Model file for the job. Use its own axes, mm. Face numbers are marked on the shaded views. A direction names the side the tool comes from. Give positions to 0.01 mm unless a question says otherwise; leave off trailing zeros. Answer in a Markdown table with one row per item.
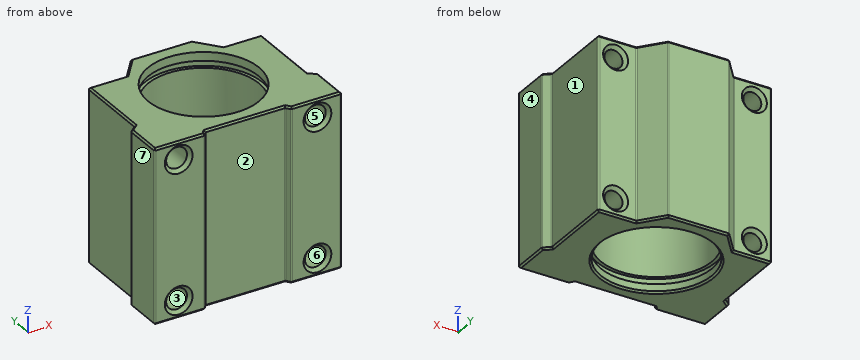
```python
from build123d import *

# Parameters (mm, degrees)
SKETCH1_R           = 16
BOSS_EXTRUDE1_DEPTH = 50
CUT_EXTRUDE1_REACH  = 72.071
SKETCH2_R           = 2.6
SKETCH3_R           = 3
CUT_EXTRUDE2_DEPTH  = 12
SKETCH4_W           = 2
SKETCH4_H           = 1
CHAMFER1_SIZE       = 1
CHAMFER2_SIZE       = 0.5
FILLET2_R           = 0.5


with BuildPart() as part:
    # Sketch1 → Boss-Extrude1 (new body)
    with BuildSketch(Plane.XY):
        Polygon((8.75, 0), (-8.75, 0), (-14, -6.5), (-25, -6.5), (-25, -28.31372549), (-27, -30), (-27, -41), (-12.5, -41), (-11.5, -39.7), (11.5, -39.7), (12.5, -41), (27, -41), (27, -30), (25, -28.31372549), (25, -6.5), (14, -6.5), align=None)
        with Locations((0, -20)):
            Circle(SKETCH1_R, mode=Mode.SUBTRACT)
    extrude(amount=BOSS_EXTRUDE1_DEPTH)

    # Sketch2 → Cut-Extrude1 (cut, up to next)
    with BuildSketch(Plane(origin=(0, 0, 0), x_dir=(1, 0, 0), z_dir=(0, 1, 0)), mode=Mode.PRIVATE) as cut_extrude1_sk1:
        with Locations(Location((-20, -45, 0), (0, 0, 270))):
            Circle(SKETCH2_R)
    cut_extrude1_tool1 = extrude(cut_extrude1_sk1.sketch, amount=-CUT_EXTRUDE1_REACH, mode=Mode.PRIVATE) & part.part
    # Sketch2 → Cut-Extrude1 (cut, up to next)
    with BuildSketch(Plane(origin=(0, 0, 0), x_dir=(1, 0, 0), z_dir=(0, 1, 0)), mode=Mode.PRIVATE) as cut_extrude1_sk2:
        with Locations(Location((20, -45, 0), (0, 0, 270))):
            Circle(SKETCH2_R)
    cut_extrude1_tool2 = extrude(cut_extrude1_sk2.sketch, amount=-CUT_EXTRUDE1_REACH, mode=Mode.PRIVATE) & part.part
    # Sketch2 → Cut-Extrude1 (cut, up to next)
    with BuildSketch(Plane(origin=(0, 0, 0), x_dir=(1, 0, 0), z_dir=(0, 1, 0)), mode=Mode.PRIVATE) as cut_extrude1_sk3:
        with Locations(Location((20, -5, 0), (0, 0, 270))):
            Circle(SKETCH2_R)
    cut_extrude1_tool3 = extrude(cut_extrude1_sk3.sketch, amount=-CUT_EXTRUDE1_REACH, mode=Mode.PRIVATE) & part.part
    # Sketch2 → Cut-Extrude1 (cut, up to next)
    with BuildSketch(Plane(origin=(0, 0, 0), x_dir=(1, 0, 0), z_dir=(0, 1, 0)), mode=Mode.PRIVATE) as cut_extrude1_sk4:
        with Locations(Location((-20, -5, 0), (0, 0, 270))):
            Circle(SKETCH2_R)
    cut_extrude1_tool4 = extrude(cut_extrude1_sk4.sketch, amount=-CUT_EXTRUDE1_REACH, mode=Mode.PRIVATE) & part.part
    add(cut_extrude1_tool1.solids().sort_by_distance((-20, 0, 45))[0], mode=Mode.SUBTRACT)
    add(cut_extrude1_tool2.solids().sort_by_distance((20, 0, 45))[0], mode=Mode.SUBTRACT)
    add(cut_extrude1_tool3.solids().sort_by_distance((20, 0, 5))[0], mode=Mode.SUBTRACT)
    add(cut_extrude1_tool4.solids().sort_by_distance((-20, 0, 5))[0], mode=Mode.SUBTRACT)

    # Sketch3 → Cut-Extrude2 (cut)
    with BuildSketch(Plane.XZ.offset(41)):
        with Locations(Location((-20, 45, 0), (0, 0, 270))):
            Circle(SKETCH3_R)
        with Locations(Location((20, 45, 0), (0, 0, 90))):
            Circle(SKETCH3_R)
        with Locations(Location((20, 5, 0), (0, 0, 270))):
            Circle(SKETCH3_R)
        with Locations(Location((-20, 5, 0), (0, 0, 90))):
            Circle(SKETCH3_R)
    extrude(amount=-CUT_EXTRUDE2_DEPTH, mode=Mode.SUBTRACT)

    # Sketch4 → Cut-Revolve1 (revolve, cut)
    with BuildSketch(Plane(origin=(0, 0, 0), x_dir=(0, 0, -1), z_dir=(1, 0, 0))):
        with Locations((-46.5, -3.5)):
            Rectangle(SKETCH4_W, SKETCH4_H)
        with Locations((-3.5, -3.5)):
            Rectangle(SKETCH4_W, SKETCH4_H)
    revolve(axis=Axis((0, -20, 0), (0, 0, 1)), mode=Mode.SUBTRACT)

    # Chamfer1
    chamfer1_edges = [part.edges().sort_by_distance(p)[0] for p in [
        (-20, -6.5, 42.4),
        (20, -6.5, 42.4),
        (20, -6.5, 2.4),
        (-20, -6.5, 2.4),
        (-20, -41, 48),
        (20, -41, 42),
        (20, -41, 8),
        (-20, -41, 2),
    ]]
    chamfer(chamfer1_edges, length=CHAMFER1_SIZE)

    # Chamfer2
    chamfer2_edges = [part.edges().sort_by_distance(p)[0] for p in [
        (0, -39.7, 50),
        (12, -40.35, 50),
        (-27, -35.5, 0),
        (-26, -29.156862745, 0),
        (-25, -17.406862745, 0),
        (-19.5, -6.5, 0),
        (-11.375, -3.25, 0),
        (19.75, -41, 50),
        (0, 0, 0),
        (11.375, -3.25, 0),
        (19.5, -6.5, 0),
        (25, -17.406862745, 0),
        (26, -29.156862745, 0),
        (27, -35.5, 0),
        (19.75, -41, 0),
        (12, -40.35, 0),
        (27, -35.5, 50),
        (0, -39.7, 0),
        (-12, -40.35, 0),
        (-19.75, -41, 0),
        (26, -29.156862745, 50),
        (25, -17.406862745, 50),
        (19.5, -6.5, 50),
        (11.375, -3.25, 50),
        (0, 0, 50),
        (-11.375, -3.25, 50),
        (-16, -20, 0),
        (-19.75, -41, 50),
        (-19.5, -6.5, 50),
        (-25, -17.406862745, 50),
        (-26, -29.156862745, 50),
        (-27, -35.5, 50),
        (-12, -40.35, 50),
    ]]
    chamfer(chamfer2_edges, length=CHAMFER2_SIZE)

    # Fillet2
    fillet2_edges = [part.edges().sort_by_distance(p)[0] for p in [
        (14, -6.5, 25),
        (25, -6.5, 25),
        (8.75, 0, 25),
        (-8.75, 0, 25),
        (-14, -6.5, 25),
        (-25, -6.5, 25),
        (-25, -28.31372549, 25),
        (-27, -30, 25),
        (-27, -41, 25),
        (-12.5, -41, 25),
        (-11.5, -39.7, 25),
        (11.5, -39.7, 25),
        (12.5, -41, 25),
        (27, -41, 25),
        (27, -30, 25),
        (25, -28.31372549, 25),
    ]]
    fillet(fillet2_edges, radius=FILLET2_R)


solid = part.part
```
(1) Which spindle directions (+Z, -Z, +X, -X, +Y, -Y) get a long thin tool onto all of the face, cutting with end or side? Do the marked faces 1, 2 and 3. Say none if no direction does.
Established:
| item | result |
|---|---|
| face 1 | +Z, -Z, +X, +Y |
| face 2 | +Z, -Z, -Y |
| face 3 | -Y |
(2) Mould opens along X. For the marked faces 4, 5, 6 and 7 say: pulls with the +X half, pulls with the -X half, needs draft (parallel to the pull), parting line crosses it, or undercut.
Established:
| item | result |
|---|---|
| face 4 | pulls with the +X half |
| face 5 | undercut |
| face 6 | undercut |
| face 7 | pulls with the -X half |
(3) Flat gauge pins, fed straight in: P1, Ø9.5, axis at x = -20, z = 45, coming from the +Y side; P2, Ø10, axis at x = 5.5, z = 38.5, coming from the -Y side; P3, Ø7, axis at x = 20, z = 5, coming from the -Y side. Where does each tip first touch, or does it go through?
Established:
| item | result |
|---|---|
| P1 | stops at y = -6.5 |
| P2 | stops at y = -39.7 |
| P3 | stops at y = -40.5 |
(4) Saw through at A-A, the plane y = -20. Count the separate pieces of the cut face and the enclosed holes in it, and give its area (3 significant figures).
Established:
| item | result |
|---|---|
| separate pieces | 2 |
| enclosed holes | 4 |
| area | 806 mm2 |
(5) Wall check: L1, parallel to Z at x = 21, y = -16; L2, parallel to Y at x = 0, z = 48.3; L3, parallel to X at y = -33, z = 5. Give the ranges that are in metal, low to high.
Established:
| item | result |
|---|---|
| L1 | z = 0 to 2.6, 7.4 to 42.6, 47.4 to 50 |
| L2 | y = -39.7 to -36, -4 to 0 |
| L3 | x = -27 to -23, -17 to -9.33, 9.33 to 17, 23 to 27 |
